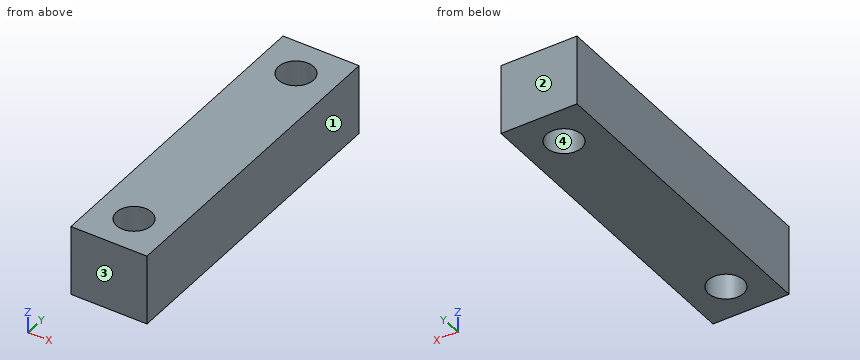
Autodesk Inventor part; units mm, degrees
ref_plane "YZ Plane" through (0, 0, 0) normal (1, 0, 0) x (0, 1, 0)
ref_plane "XZ Plane" through (0, 0, 0) normal (0, 1, 0) x (-1, 0, 0)
ref_plane "XY Plane" through (0, 0, 0) normal (0, 0, 1) x (1, 0, 0)
sketch "Sketch1" plane through (0, 0, 0) normal (0, 0, 1) x (1, 0, 0)
  line L0 (0, 55) -> (13, 55)
  line L1 (13, 55) -> (13, 0)
  line L2 (13, 0) -> (0, 0)
  line L3 (0, 0) -> (0, 55)
  circle A0 centre (6.5, 48.5) radius 3
  circle A1 centre (6.5, 6.5) radius 3
  line L4 (6.5, 48.5) -> (6.5, 6.5)
  dimension "d2" = 6
  dimension "d3" = 6
  dimension "d4" = 42
  dimension "d5" = 55
  dimension "d6" = 13
  dimension "d7" = 6.5
  dimension "d8" = 6.5
extrude "Extrusion1" add sketch "Sketch1" along normal blind 12
equation "\"d3\" = d2"
equation "\"d7\" = 0.5 * d6"
equation "\"d8\" = -0.5 * d4 + 0.5 * d5"
properties part number "plateplummer" material "PMMA Plastic"
Geometry: final body of the model. Coordinates: model frame, mm. Face numbers are marked on the shaded views. Round coordinates to 2 decimals unless told otherwise and drop trailing zeros. Loops run counter-clockwise (first coordinate to the right, second up) from the corner with the lowest first, then second, coordinate; pieces in that order, holes last. Notation, with made-up numbers: M -13,41.25 L 11,41.25 A22 cw 11,73.25 Z; hole C 49,-29.5 d10. An arc over 180 degrees is marked long. Put each result on its own line as item: value. Start each with the question number.
(1) Contact query for flat-ended pins moving along their axis: pin 1 Ø3 at (y, z) = (9, 9.5) entering from -X; pin 2 Ø3.5 at (x, y) = (6.5, 48.5) entering from -Z (1 decimal). Output: stop coordinate, or through.
(2) Material intervals for line 1 along Y through (x, z) = (6.5, 9); line 2 along X through (y, z) = (6.5, 5.75); line 3 along Y through (x, z) = (8.75, 4.5), sorted ascending. Write a range as [from, to].
(3) Section query B-B (x = 6.5). Return loops of the section in (y, z).
(4) Draft query along Y for the marked faces 1, 2, 3 and 4. Return one class per face: +Y half, -Y half, draft (parallel to the pull), parting line (faces both ways), or undercut.
(5) Section query C-C (z = 1.25). Return loops of the section in (x, y), then the cut area to 3 significant figures.
(6) Section query A-A (y = 48.5). Return loops of the section in (x, z), then the cut area to 3 significant figures.
Findings below:
1. pin 1: stops at x = 0
1. pin 2: passes through
2. line 1: y = [0, 3.5], [9.5, 45.5], [51.5, 55]
2. line 2: x = [0, 3.5], [9.5, 13]
2. line 3: y = [0, 4.52], [8.48, 46.52], [50.48, 55]
3. outline: M 0,0 L 3.5,0 L 3.5,12 L 0,12 Z; M 9.5,0 L 45.5,0 L 45.5,12 L 9.5,12 Z; M 51.5,0 L 55,0 L 55,12 L 51.5,12 Z
4. face 1: draft
4. face 2: +Y half
4. face 3: -Y half
4. face 4: undercut
5. outline: M 0,0 L 13,0 L 13,55 L 0,55 Z; hole C 6.5,6.5 d6; hole C 6.5,48.5 d6
5. area: 658 mm2
6. outline: M 0,0 L 3.5,0 L 3.5,12 L 0,12 Z; M 9.5,0 L 13,0 L 13,12 L 9.5,12 Z
6. area: 84.0 mm2
